Source: CAD feature listing. Evaluate the final solid. Frame: model axes, mm. A direction names the side the tool comes from. Coordinates: 2 decimals unless noted, no trailing zeros. Order: outer loops, then holes, each group sorted by start corner. A loop starts at its lowest first (then second) coordinate and runs counter-clockwise, first axis right, second up. Notation, with made-up numbers: (-19, 63.25) -> (17, 63.25) arc R32 ccw to (17, 93.25) -> close; hole circle Ø7 at (42, -24). An arc over 180 degrees is marked (long way). Put each result on its own line as item: value.
from build123d import *

# Parameters (mm, degrees)
SKETCH1_W                      = 180
SKETCH1_H                      = 10
BOSS_EXTRUDE1_DEPTH            = 10
SKETCH2_W                      = 10
SKETCH2_H                      = 10
BOSS_EXTRUDE2_DEPTH            = 140
M5_CLEARANCE_HOLE1_D           = 5.5
M5_CLEARANCE_HOLE1_CSINK_D     = 5.55
M5_CLEARANCE_HOLE1_CSINK_ANGLE = 90
BOSS_EXTRUDE3_START            = 2.5
BOSS_EXTRUDE3_DEPTH            = 10
HOLE1_D                        = 10.2
HOLE1_DEPTH                    = 10
HOLE1_CBORE_D                  = 11.4
HOLE1_CBORE_DEPTH              = 0.6


with BuildPart() as part:
    # Sketch1 → Boss-Extrude1 (new body)
    with BuildSketch(Plane(origin=(0, 0, 0), x_dir=(1, 0, 0), z_dir=(0, 1, 0))):
        Rectangle(SKETCH1_W, SKETCH1_H)
    extrude(amount=BOSS_EXTRUDE1_DEPTH)

    # Sketch2 → Boss-Extrude2 (add)
    with BuildSketch(Plane(origin=(0, 10, 0), x_dir=(1, 0, 0), z_dir=(0, 1, 0))):
        with Locations((-85, 0)):
            Rectangle(SKETCH2_W, SKETCH2_H)
        with Locations((85, 0)):
            Rectangle(SKETCH2_W, SKETCH2_H)
    extrude(amount=BOSS_EXTRUDE2_DEPTH)

    # M5 Clearance Hole1 (through all)
    with Locations(Plane(origin=(90, 0, 0), x_dir=(0, 0, -1), z_dir=(1, 0, 0))):
        with Locations((0, 145)):
            CounterSinkHole(M5_CLEARANCE_HOLE1_D / 2, M5_CLEARANCE_HOLE1_CSINK_D / 2, counter_sink_angle=M5_CLEARANCE_HOLE1_CSINK_ANGLE)

    # Sketch6 → Boss-Extrude3 (add)
    with BuildSketch(Plane(origin=(0, 0, 0), x_dir=(0, 0, -1), z_dir=(1, 0, 0)).offset(BOSS_EXTRUDE3_START)):
        Polygon((5, 0), (5, 10), (-5, 10), (-5, 30), (15, 30), (15, 0), align=None)
    extrude(amount=BOSS_EXTRUDE3_DEPTH)

    # Hole1
    with Locations(Plane.ZY.offset(-2.5)):
        with Locations((-5, 20)):
            CounterBoreHole(HOLE1_D / 2, HOLE1_CBORE_D / 2, HOLE1_CBORE_DEPTH, depth=HOLE1_DEPTH)


solid = part.part
1. Cut plane A-A on y = 20. Output: boundary loops of the cut face in (x, z), plus the area to 3 significant figures.
Numbers:
outline: (-90, -5) -> (-80, -5) -> (-80, 5) -> (-90, 5) -> close; (2.5, -15) -> (12.5, -15) -> (12.5, -10.1) -> (3.1, -10.1) -> (3.1, -10.7) -> (2.5, -10.7) -> close; (2.5, 0.7) -> (3.1, 0.7) -> (3.1, 0.1) -> (12.5, 0.1) -> (12.5, 5) -> (2.5, 5) -> close; (80, -5) -> (90, -5) -> (90, 5) -> (80, 5) -> close
area: 297 mm2
2. Ray query, line 1 along X through (y, z) = (17, -0.5); line 2 along Y through (x, z) = (2.9, -5); line 3 along Y through (x, z) = (-87.75, 0). Return the intervals inside material, ascending.
Numbers:
line 1: x = -90 to -80, 3.1 to 12.5, 80 to 90
line 2: y = 0 to 14.3, 25.7 to 30
line 3: y = 0 to 142.25, 147.75 to 150
3. First-contact query: pin 1 (3.5 mm diameter, centred on y = 145, z = 0, fed in from -X); pin 2 (12 mm diameter, centred on y = 102.5, z = -6.5, fed in from -X); pin 3 (8 mm diameter, centred on x = 6.5, z = -6, fed in from +Y); pin 4 (11 mm diameter, centred on x = -45, z = -0.5, fed in from +Y). Flat tips, straight axial feed; report the tip coordinate or a pass-through.
Numbers:
pin 1: passes through
pin 2: stops at x = -90
pin 3: stops at y = 30
pin 4: stops at y = 10
4. Cut plane B-B on y = 111.5. Output: boundary loops of the cut face in (x, z), plus the area to 3 significant figures.
Numbers:
outline: (-90, -5) -> (-80, -5) -> (-80, 5) -> (-90, 5) -> close; (80, -5) -> (90, -5) -> (90, 5) -> (80, 5) -> close
area: 200 mm2
5. Cut plane D-D on x = 34.5. Output: boundary loops of the cut face in (y, z), plus the area to 3 significant figures.
Numbers:
outline: (0, -5) -> (10, -5) -> (10, 5) -> (0, 5) -> close
area: 100 mm2
6. Set-up query: faces 1 (the flat face through (-80, 79, 0)), 2 (the flat face through (12.5, 15, -7)), 3 (the cylindrical face through (8, 15, -4)). Return all of +Z, -Z, +X, -X, +Y, -Y with unobstructed straight access to the full face (end or side cutting, diameter ignored); none if empty.
Numbers:
face 1: +Z, -Z, +Y
face 2: -Z, +Y
face 3: none
7. Pull-direction query (X, two-part tool) for faces 4 (the flat face through (-90, 74, 0)), 5 (the flat face through (90, 74, 0)), 6 (the flat face through (80, 79, 0)), 7 (the flat face through (-1, 0, -1)); classes: pulls with the +X half, pulls with the -X half, needs draft (parallel to the pull), parting line crosses it, or undercut.
Numbers:
face 4: pulls with the -X half
face 5: pulls with the +X half
face 6: undercut
face 7: needs draft
8. Cut plane C-C on y = 145. Output: boundary loops of the cut face in (x, z) (3 decimals), plus the area to 3 significant figures.
Numbers:
outline: (-90, -5) -> (-80, -5) -> (-80, -2.75) -> (-90, -2.75) -> close; (-90, 2.75) -> (-80, 2.75) -> (-80, 5) -> (-90, 5) -> close; (80, -5) -> (90, -5) -> (90, -2.775) -> (89.975, -2.75) -> (80, -2.75) -> close; (80, 2.75) -> (89.975, 2.75) -> (90, 2.775) -> (90, 5) -> (80, 5) -> close
area: 90.0 mm2
